CAD build for the part. Positions are in the model's coordinates, mm. A direction names the side the tool comes from. Give positions to 0.01 mm unless a question says otherwise; leave off trailing zeros. Loops run counter-clockwise (first coordinate to the right, second up) from the corner with the lowest first, then second, coordinate; pieces in that order, holes last.
```python
from build123d import *

# Parameters (mm, degrees)
SKETCH1_W               = 85
SKETCH1_H               = 55
BOSS_EXTRUDE2_DEPTH     = 3
CUT_EXTRUDE1_DEPTH      = 51.709959574
CUT_EXTRUDE1_DEPTH_BACK = 51.709959574
SKETCH3_W               = 27
SKETCH3_H               = 25
FILLET2_R               = 10
SKETCH4_R               = 8
BOSS_EXTRUDE3_DEPTH     = 3
FILLET3_R               = 10
CUT_EXTRUDE2_DEPTH      = 62.072254936
CUT_EXTRUDE2_DEPTH_BACK = 62.072254936
CUT_EXTRUDE3_DEPTH      = 62.072255079
CUT_EXTRUDE3_DEPTH_BACK = 62.072255079
SKETCH6_R               = 1.5


with BuildPart() as part:
    # Sketch1 → Boss-Extrude2 (new body)
    with BuildSketch(Plane.XY):
        Rectangle(SKETCH1_W, SKETCH1_H)
    extrude(amount=BOSS_EXTRUDE2_DEPTH)

    # Sketch3 → Cut-Extrude1 (cut, two sides: drawn at the far end of the back side and taken through both)
    with BuildSketch(Plane.XY.offset(3).offset(-CUT_EXTRUDE1_DEPTH_BACK)):
        with Locations((-19.5, 9)):
            Rectangle(SKETCH3_W, SKETCH3_H)
        with Locations((19.5, 9)):
            Rectangle(SKETCH3_W, SKETCH3_H)
    extrude(amount=CUT_EXTRUDE1_DEPTH + CUT_EXTRUDE1_DEPTH_BACK, mode=Mode.SUBTRACT)

    # Fillet2
    fillet2_edges = [part.edges().sort_by_distance(p)[0] for p in [
        (-42.5, -27.5, 1.5),
        (42.5, -27.5, 1.5),
    ]]
    fillet(fillet2_edges, radius=FILLET2_R)

    # Sketch4 → Boss-Extrude3 (add)
    with BuildSketch(Plane.XY):
        with Locations((-43.301270189, 25)):
            Circle(SKETCH4_R)
        with Locations((43.301270189, 25)):
            Circle(SKETCH4_R)
    extrude(amount=BOSS_EXTRUDE3_DEPTH)

    # Fillet3
    fillet3_edges = [part.edges().sort_by_distance(p)[0] for p in [
        (-35.701928112, 27.5, 1.5),
        (-42.5, 17.040228264, 1.5),
        (35.701928112, 27.5, 1.5),
        (42.5, 17.040228264, 1.5),
    ]]
    fillet(fillet3_edges, radius=FILLET3_R)

    # Sketch5 → Cut-Extrude2 (cut, two sides: drawn at the far end of the back side and taken through both)
    with BuildSketch(Plane.XY.offset(3).offset(-CUT_EXTRUDE2_DEPTH_BACK)):
        with BuildLine():
            Line((-14.657223741, -11.118605282), (15.937497294, -10.788446422))
            add(Edge.make_bspline(
                [(-14.657223741, -11.118605282), (-18.533826982, -14.187506868), (7.467986251, -17.149664061), (15.801657819, -10.897471716), (15.937497294, -10.788446422)],
                knots=[0, 0, 0, 0, 0.49190671, 0.50088311, 0.50088311, 0.50088311, 0.50088311], degree=3))
        make_face()
    extrude(amount=CUT_EXTRUDE2_DEPTH + CUT_EXTRUDE2_DEPTH_BACK, mode=Mode.SUBTRACT)

    # Sketch6 → Cut-Extrude3 (cut, two sides: drawn at the far end of the back side and taken through both)
    with BuildSketch(Plane.XY.offset(3).offset(-CUT_EXTRUDE3_DEPTH_BACK)):
        with Locations((-6, -23.5)):
            Circle(SKETCH6_R)
        with Locations((6, -23.5)):
            Circle(SKETCH6_R)
    extrude(amount=CUT_EXTRUDE3_DEPTH + CUT_EXTRUDE3_DEPTH_BACK, mode=Mode.SUBTRACT)


solid = part.part
```
1. Saw through at D-D, the plane z = 0.55. Count the separate pieces of the cut face and the enclosed holes in it, and give its area (3 significant figures).
Responses:
separate pieces: 1
enclosed holes: 5
area: 3,480 mm2
2. Saw through at C-C, the plane y = 2. List the corners of the cut face in (x, z).
Responses:
outline: (-42.5, 0) - (-33, 0) - (-33, 3) - (-42.5, 3) - close; (-6, 0) - (6, 0) - (6, 3) - (-6, 3) - close; (33, 0) - (42.5, 0) - (42.5, 3) - (33, 3) - close
3. Drop flat-ended pins along their axis: pin 1 (1.8 mm diameter, centred on x = -6, y = -23.5, fed in from +Z); pin 2 (0.9 mm diameter, centred on y = -9.5, z = 2, fed in from +X); pin 3 (1.5 mm diameter, centred on y = 3.5, z = 1, fed in from -X); pin 4 (0.9 mm diameter, centred on x = -9, z = 1, fed in from +Y). Give the stop position or say it passes through.
Responses:
pin 1: passes through
pin 2: stops at x = 42.5
pin 3: stops at x = -42.5
pin 4: stops at y = 27.5
4. Pull direction Y, two halves, no side cores. Call faces 4 (the face through (0, 27.5, 1)), 5 (the face through (-42.5, -4, 1)), 6 (the face through (19, 21.5, 1)), 7 (the face through (-49.453, 30.115, 1.479)): released by +Y, released by -Y, zero draft, split by the parting line, or undercut.
Responses:
face 4: released by +Y
face 5: zero draft
face 6: undercut
face 7: split by the parting line
5. Saw through at B-B, the plane x = 24.5. List the corners of the cut face in (y, z).
Responses:
outline: (-27.5, 0) - (-3.5, 0) - (-3.5, 3) - (-27.5, 3) - close; (21.5, 0) - (27.5, 0) - (27.5, 3) - (21.5, 3) - close
6. Tool access for faces 1 (the face through (-34.206, 28.274, 1.479)), 2 (the face through (-43.772, 14.409, 1.479)), 3 (the face through (6, 9, 1)): list every direction of +Z, -Z, +X, -X, +Y, -Y with a clear straight run to the whole face (end or side of a thin tool).
Responses:
face 1: +Z, -Z, +Y
face 2: +Z, -Z, -X, -Y
face 3: +Z, -Z
7. Probe line 1 along X through (y, z) = (9, 1.55); line 2 along X through (y, z) = (-23.5, 1.05); line 3 along Y through (x, z) = (-7, 2.2). List the from-to ranges inside material, lowest first.
Responses:
line 1: x = -42.5 to -33, -6 to 6, 33 to 42.5
line 2: x = -40.5 to -7.5, -4.5 to 4.5, 7.5 to 40.5
line 3: y = -27.5 to -24.62, -22.38 to -14.3, -11.04 to -3.5, 21.5 to 27.5
8. Saw through at A-A, the plane y = -23.5. List the corners of the cut face in (x, z), and give its area (3 significant figures).
Responses:
outline: (-40.5, 0) - (-7.5, 0) - (-7.5, 3) - (-40.5, 3) - close; (-4.5, 0) - (4.5, 0) - (4.5, 3) - (-4.5, 3) - close; (7.5, 0) - (40.5, 0) - (40.5, 3) - (7.5, 3) - close
area: 225 mm2
